Model file for the job. Use its own axes, mm. A direction names the side the tool comes from. Round coordinates to 2 decimals unless told otherwise and drop trailing zeros. Order: outer loops, then holes, each group sorted by start corner. A loop starts at its lowest first (then second) coordinate and runs counter-clockwise, first axis right, second up. Notation, with made-up numbers: M 0,-4.5 L 11,-4.5 A23 ccw 11,12.5 Z; hole C -28.75,36.25 d9. An arc over 180 degrees is marked long. Return JSON: item names as keys, results as strings. Group by question number.
Item 1: Slice it at D-D on y = -18.5. Write the cut outline in (x, z).
Item 2: Pull direction Y, two halves, no side cores. Call faces 1 (the face through (18.5, 94, -0.1)), 2 (the face through (19.88, -19.72, -1.08)), 3 (the face through (19.88, 85.76, 6.06)): pulls with the +Y half, pulls with the -Y half, needs draft (parallel to the pull), parting line crosses it, or undercut.
Item 3: Pin check, flat tips, straight feed: pin 1 Ø10 at (y, z) = (51, 0) entering from +X; pin 2 Ø12 at (y, z) = (68.5, -3.5) entering from +X; pin 3 Ø8 at (y, z) = (81.5, -3.5) entering from +X. Stop position of each tip, or through.
Item 4: Slice it at B-B on x = 8.75. Give the number of separate pieces and of enclosed holes in the cut face, then the cut area to 3 significant figures.
Item 5: Slice it at A-A on y = 76. Write the cut outline in (x, z), then the cut area to 3 significant figures.
Item 6: Which spindle directions (+Z, -Z, +X, -X, +Y, -Y) get a long thin tool onto all of the face, cutting with end or side? Do faces 4 (the face through (17, 85, 0)), 5 (the face through (19.9, 39.2, -5.9)), 6 (the face through (5.472, 49.053, -2.539)). Say none if no direction does.
Item 7: Probe line 1 along Y through (x, z) = (5, 0); line 2 along Z through (x, y) = (8.75, 76); line 3 along Y through (x, z) = (2.5, 2). List the from-to ranges inside material, lowest first.
from build123d import *

# Parameters (mm, degrees)
DODANIE_WYCI_GNI_CIE1_DEPTH                        = 100
SFAZOWANIE1_SIZE                                   = 10
ZAOKR_GLENIE1_R                                    = 10
SZKIC3_W                                           = 20
SZKIC3_H                                           = 45
WYTNIJ_WYCI_GNI_CIE1_DEPTH                         = 100
SFAZOWANIE2_SIZE2                                  = 0.890457371
SFAZOWANIE2_SIZE                                   = 2
SFAZOWANIE3_SIZE2                                  = 0.727940469
SFAZOWANIE3_SIZE                                   = 2
POG_BIENIE_STO_KOWE_POD_M6_WKR_T_Z_BEM_D           = 6.4
POG_BIENIE_STO_KOWE_POD_M6_WKR_T_Z_BEM_DEPTH       = 40
POG_BIENIE_STO_KOWE_POD_M6_WKR_T_Z_BEM_CSINK_D     = 13.44
POG_BIENIE_STO_KOWE_POD_M6_WKR_T_Z_BEM_CSINK_ANGLE = 90
POG_BIENIE_STO_KOWE_POD_M6_WKR_T_Z_BEM_TIP         = 1.922753981
SZKIC7_R                                           = 5
DODANIE_WYCI_GNI_CIE2_DEPTH                        = 45
SFAZOWANIE5_SIZE                                   = 5
SFAZOWANIE5_SIZE2                                  = 1.819851171


with BuildPart() as part:
    # Szkic2 → Dodanie-wyciągnięcie1 (new body)
    with BuildSketch(Plane(origin=(0, 0, 0), x_dir=(1, 0, 0), z_dir=(0, 1, 0))):
        Polygon((2.12, 10), (22.5, 10), (22.5, -10), (2.12, -10), (0, -10), (0, 10), align=None)
    extrude(amount=DODANIE_WYCI_GNI_CIE1_DEPTH)

    # Sfazowanie1
    sfazowanie1_edges = [part.edges().sort_by_distance(p)[0] for p in [
        (11.25, 100, -10),
        (22.5, 100, 0),
        (11.25, 100, 10),
    ]]
    chamfer(sfazowanie1_edges, length=SFAZOWANIE1_SIZE - 0.0001)  # a hair under: the kernel refuses the full size

    # Zaokrąglenie1
    zaokr_glenie1_edges = [part.edges().sort_by_distance(p)[0] for p in [
        (22.5, 45.00005, -10),
        (22.5, 45.00005, 10),
    ]]
    fillet(zaokr_glenie1_edges, radius=ZAOKR_GLENIE1_R - 0.0001)  # a hair under: the kernel refuses the full size

    # Szkic3 → Wytnij-wyciągnięcie1 (cut)
    with BuildSketch(Plane(origin=(14.62, 0, 0), x_dir=(0, 0, -1), z_dir=(1, 0, 0))):
        with Locations((0, 62.5)):
            Rectangle(SZKIC3_W, SZKIC3_H)
    extrude(amount=WYTNIJ_WYCI_GNI_CIE1_DEPTH, mode=Mode.SUBTRACT)

    # Sfazowanie2
    sfazowanie2_edges = [part.edges().sort_by_distance(p)[0] for p in [
        (20.28459703, 40, -6.277010546),
        (20.28459703, 40, 6.277010546),
    ]]
    chamfer(sfazowanie2_edges, length=SFAZOWANIE2_SIZE, length2=SFAZOWANIE2_SIZE2)

    # Sfazowanie3
    sfazowanie3_edges = [part.edges().sort_by_distance(p)[0] for p in [
        (20.28459703, 85, -6.277010546),
        (20.28459703, 85, 6.277010546),
    ]]
    chamfer(sfazowanie3_edges, length=SFAZOWANIE3_SIZE, length2=SFAZOWANIE3_SIZE2)

    # Pogłębienie stożkowe pod M6 Wkręt z łbem stożkowym płaskim2
    with Locations(Plane(origin=(14.62, 0, 0), x_dir=(0, 0, -1), z_dir=(1, 0, 0))):
        with Locations((0, 51), (0, 76)):
            CounterSinkHole(POG_BIENIE_STO_KOWE_POD_M6_WKR_T_Z_BEM_D / 2, POG_BIENIE_STO_KOWE_POD_M6_WKR_T_Z_BEM_CSINK_D / 2, depth=POG_BIENIE_STO_KOWE_POD_M6_WKR_T_Z_BEM_DEPTH, counter_sink_angle=POG_BIENIE_STO_KOWE_POD_M6_WKR_T_Z_BEM_CSINK_ANGLE)
            with Locations((0, 0, -(POG_BIENIE_STO_KOWE_POD_M6_WKR_T_Z_BEM_DEPTH + POG_BIENIE_STO_KOWE_POD_M6_WKR_T_Z_BEM_TIP / 2))):  # 118° drill point
                Cone(0, POG_BIENIE_STO_KOWE_POD_M6_WKR_T_Z_BEM_D / 2, POG_BIENIE_STO_KOWE_POD_M6_WKR_T_Z_BEM_TIP, mode=Mode.SUBTRACT)

    # Szkic7 → Dodanie-wyciągnięcie2 (add)
    with BuildSketch(Plane.XZ):
        with Locations(Location((15, 0, 0), (0, 0, 90))):
            Circle(SZKIC7_R)
    extrude(amount=DODANIE_WYCI_GNI_CIE2_DEPTH)

    # Sfazowanie5
    sfazowanie5_edges = [part.edges().sort_by_distance(p)[0] for p in [
        (15, -45, -5),
    ]]
    sfazowanie5_side = [part.faces().sort_by_distance(p)[0] for p in [
        (15, -22.5, -5),
    ]]
    chamfer(sfazowanie5_edges, length=SFAZOWANIE5_SIZE, length2=SFAZOWANIE5_SIZE2, reference=sfazowanie5_side[0])


solid = part.part
Output values:
{
 "1": {"outline": "C 15,0 d10"},
 "2": {"face 1": "pulls with the +Y half", "face 2": "needs draft", "face 3": "undercut"},
 "3": {"pin 1": "x = 12.9", "pin 2": "x = 14.62", "pin 3": "x = 21.64"},
 "4": {"separate pieces": "1", "enclosed holes": "2", "area": "1,840 mm²"},
 "5": {"outline": "M 0,-10 L 12.5,-10 A10 ccw 14.62,-9.77 L 14.62,-6.72 L 11.1,-3.2 L 0,-3.2 Z; M 0,3.2 L 11.1,3.2 L 14.62,6.72 L 14.62,9.77 A10 ccw 12.5,10 L 0,10 Z", "area": "186 mm²"},
 "6": {"face 4": "+Z, -Z, +X", "face 5": "-Z, +X", "face 6": "+X, -X"},
 "7": {"line 1": "0 to 47.8, 54.2 to 72.8, 79.2 to 100", "line 2": "-10 to -3.2, 3.2 to 10", "line 3": "0 to 48.5, 53.5 to 73.5, 78.5 to 98"}
}
